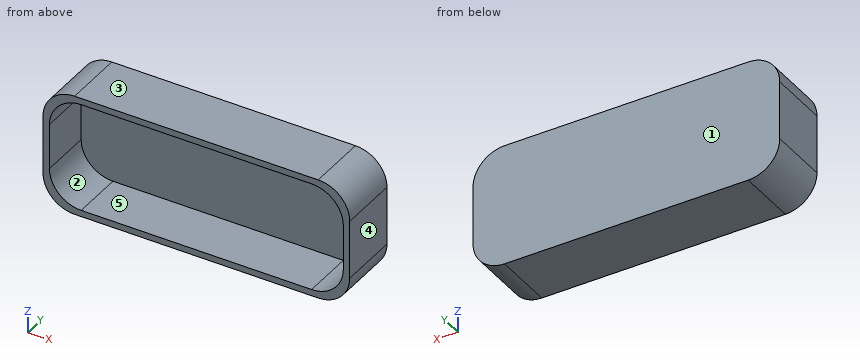
from build123d import *

# Parameters (mm, degrees)
SKETCH1_W           = 431.8
SKETCH1_H           = 171.45
BOSS_EXTRUDE1_DEPTH = 85.725
CUT_EXTRUDE1_DEPTH  = 73.025
FILLET3_R           = 44.45


with BuildPart() as part:
    # Sketch1 → Boss-Extrude1 (new body)
    with BuildSketch(Plane(origin=(0, 0, 0), x_dir=(1, 0, 0), z_dir=(0, 1, 0))):
        Rectangle(SKETCH1_W, SKETCH1_H)
    extrude(amount=BOSS_EXTRUDE1_DEPTH)

    # Sketch2 → Cut-Extrude1 (cut)
    with BuildSketch(Plane.XZ):
        with BuildLine():
            Line((162.16885638, 76.686434381), (-162.16885638, 76.686434381))
            ThreePointArc((-162.16885638, 76.686434381), (-193.771281353, 63.596281353), (-206.861434381, 31.99385638))
            Line((-206.861434381, 31.99385638), (-206.861434381, -31.99385638))
            ThreePointArc((-206.861434381, -31.99385638), (-193.771281353, -63.596281353), (-162.16885638, -76.686434381))
            Line((-162.16885638, -76.686434381), (162.16885638, -76.686434381))
            ThreePointArc((162.16885638, -76.686434381), (193.771281353, -63.596281353), (206.861434381, -31.99385638))
            Line((206.861434381, -31.99385638), (206.861434381, 31.99385638))
            ThreePointArc((206.861434381, 31.99385638), (193.771281353, 63.596281353), (162.16885638, 76.686434381))
        make_face()
    extrude(amount=-CUT_EXTRUDE1_DEPTH, mode=Mode.SUBTRACT)

    # Fillet3
    fillet3_edges = [part.edges().sort_by_distance(p)[0] for p in [
        (215.9, 42.8625, 85.725),
        (-215.9, 42.8625, 85.725),
        (-215.9, 42.8625, -85.725),
        (215.9, 42.8625, -85.725),
    ]]
    fillet(fillet3_edges, radius=FILLET3_R)


solid = part.part
Could you check a few things on this model? Use its own coordinates, in mm. Face numbers are marked on the shaded views. A direction names the side the tool comes from. Give positions to 0.01 mm unless a question says otherwise; leave off trailing zeros. Order: outer loops, then holes, each group sorted by start corner. A loop starts at its lowest first (then second) coordinate and runs counter-clockwise, first axis right, second up. Notation, with made-up numbers: (-15, 19) -> (34, 19) arc R21 ccw to (34, 58) -> close; hole circle Ø2 at (88, 28). An arc over 180 degrees is marked (long way). Return JSON: item names as keys, results as strings.
1. Thinking about a two-plate mould opening in Z: for the marked faces 3, 4 and 5, which applies, pulls with the +Z half, pulls with the -Z half, needs draft (parallel to the pull), parting line crosses it, or undercut?
Answer list:
{"face 3": "pulls with the +Z half", "face 4": "needs draft", "face 5": "undercut"}
2. Imagine slicing it at A-A on y = 27. List the corners of the cut face in (x, z) for me (3 decimals), then the cut area to 3 significant figures.
Answer list:
{"outline": "(-215.9, -41.275) arc R44.45 ccw to (-171.45, -85.725) -> (171.45, -85.725) arc R44.45 ccw to (215.9, -41.275) -> (215.9, 41.275) arc R44.45 ccw to (171.45, 85.725) -> (-171.45, 85.725) arc R44.45 ccw to (-215.9, 41.275) -> close; hole (-206.861, -31.994) arc R44.693 ccw to (-162.169, -76.686) -> (162.169, -76.686) arc R44.693 ccw to (206.861, -31.994) -> (206.861, 31.994) arc R44.693 ccw to (162.169, 76.686) -> (-162.169, 76.686) arc R44.693 ccw to (-206.861, 31.994) -> close", "area": "10,600 mm2"}
3. On a 3-axis mill with a long thin cutter (end or side, diameter ignored), from which of +Z, -Z, +X, -X, +Y, -Y can I reach the whole of each face in a straight line? I mean the marked faces 1 and 2. Say none if no direction works.
Answer list:
{"face 1": "+Z, -Z, +X, -X, +Y", "face 2": "-Y"}
4. Imagine slicing it at B-B on x = -149.5. List the corners of the cut face in (y, z) for me (3 decimals), then the cut area to 3 significant figures.
Answer list:
{"outline": "(0, -85.725) -> (85.725, -85.725) -> (85.725, 85.725) -> (0, 85.725) -> (0, 76.686) -> (73.025, 76.686) -> (73.025, -76.686) -> (0, -76.686) -> close", "area": "3,500 mm2"}
5. I need wall thicknesses on line 1 (Z direction, x = 48, y = 59) (3 decimals); line 2 (X direction, y = 30.5, z = 13); line 3 (Y direction, x = -119, z = -3.5) (3 decimals). Which ranges of each line are inside material? Lowest first, please. Write a range as from..to.
Answer list:
{"line 1": "z = -85.725..-76.686, 76.686..85.725", "line 2": "x = -215.9..-206.86, 206.86..215.9", "line 3": "y = 73.025..85.725"}
6. For pin 1 Ø2 at (x, z) = (80, -60.5) entering from -Y (3 decimals), with a flat end and sliding along its axis, tell me the tip position at first contact or that it passes through.
Answer list:
{"pin 1": "stops at y = 73.025"}
7. Imagine slicing it at C-C on z = -2. List the corners of the cut face in (x, y) for me (3 decimals).
Answer list:
{"outline": "(-215.9, 0) -> (-206.861, 0) -> (-206.861, 73.025) -> (206.861, 73.025) -> (206.861, 0) -> (215.9, 0) -> (215.9, 85.725) -> (-215.9, 85.725) -> close"}
